```python
from build123d import *

# Parameters (mm, degrees)
BOSS_EXTRU_1_DEPTH      = 1380
ENL_V_MAT_EXTRU_1_DEPTH = 70


with BuildPart() as part:
    # Esquisse2 → Boss.-Extru.1 (new body)
    with BuildSketch(Plane.XY):
        with BuildLine():
            Line((2, 0), (38, 0))
            ThreePointArc((38, 0), (39.414213562, 0.585786438), (40, 2))
            Line((40, 2), (40, 38))
            ThreePointArc((40, 38), (39.414213562, 39.414213562), (38, 40))
            Line((38, 40), (2, 40))
            ThreePointArc((2, 40), (0.585786438, 39.414213562), (0, 38))
            Line((0, 38), (0, 2))
            ThreePointArc((0, 2), (0.585786438, 0.585786438), (2, 0))
        make_face()
        with BuildLine():
            Line((6, 4), (34, 4))
            ThreePointArc((34, 4), (35.414213562, 4.585786438), (36, 6))
            Line((36, 6), (36, 34))
            ThreePointArc((36, 34), (35.414213562, 35.414213562), (34, 36))
            Line((34, 36), (6, 36))
            ThreePointArc((6, 36), (4.585786438, 35.414213562), (4, 34))
            Line((4, 34), (4, 6))
            ThreePointArc((4, 6), (4.585786438, 4.585786438), (6, 4))
        make_face(mode=Mode.SUBTRACT)
    extrude(amount=BOSS_EXTRU_1_DEPTH)

    # Esquisse3 → Enlèv. mat.-Extru.1 (cut)
    with BuildSketch(Plane(origin=(0, 40, 0), x_dir=(1, 0, 0), z_dir=(0, 1, 0))):
        Polygon((0, -1380), (40, -1340), (40, -1380), align=None)
    extrude(amount=-ENL_V_MAT_EXTRU_1_DEPTH, mode=Mode.SUBTRACT)


solid = part.part
```
Check sheet for the modelled part. Datum: model origin and axes. Units: mm. A direction names the side the tool comes from. Give positions to 0.01 mm unless a question says otherwise; leave off trailing zeros. Order: outer loops, then holes, each group sorted by start corner. A loop starts at its lowest first (then second) coordinate and runs counter-clockwise, first axis right, second up. Notation, with made-up numbers: M 11.5,27.5 L 61.5,27.5 A33 ccw 61.5,58.5 Z; hole C 58,61.5 d5. An arc over 180 degrees is marked long. Answer in a Markdown table with one row per item.
1) Access from +Z, -Z, +X, -X, +Y, -Y to the whole of each face (thin tool, end or side, straight path). Record for faces 1 (the flat face through (4, 20, 678)), 2 (the flat face through (40, 20, 661)).
Filled sheet:
| item | result |
|---|---|
| face 1 | +Z, -Z |
| face 2 | +Z, -Z, +X, +Y, -Y |
2) Release check for a two-part mould opening along Y. For faces 3 (the flat face through (20, 4, 677)), 4 (the flat face through (36, 20, 663)), 5 (the flat face through (20, 0, 679)), 6 (the flat face through (20, 3, 1360)) record: +Y half, -Y half, draft (parallel to the pull), parting line (faces both ways), or undercut.
Filled sheet:
| item | result |
|---|---|
| face 3 | undercut |
| face 4 | undercut |
| face 5 | -Y half |
| face 6 | draft |
3) Thickness scan on L1, parallel to X at y = 6.5, z = 839.5; L2, parallel to Z at x = 2, y = 24.5. Record the ranges inside material, lowest first. Write a range as [from, to].
Filled sheet:
| item | result |
|---|---|
| L1 | x = [0, 4], [36, 40] |
| L2 | z = [0, 1378] |
4) Cross-section at A-A, the plane x = 17. Enter the section's corners in (y, z).
Filled sheet:
| item | result |
|---|---|
| outline | M 0,0 L 4,0 L 4,1363 L 0,1363 Z; M 36,0 L 40,0 L 40,1363 L 36,1363 Z |
5) Cross-section at B-B, the plane y = 19.5. Enter the section's corners in (x, z).
Filled sheet:
| item | result |
|---|---|
| outline | M 0,0 L 4,0 L 4,1376 L 0,1380 Z; M 36,0 L 40,0 L 40,1340 L 36,1344 Z |
6) Cross-section at C-C, the plane z = 1127.5. Enter the section's corners in (x, y), plus the area to 3 significant figures.
Filled sheet:
| item | result |
|---|---|
| outline | M 0,2 A2 ccw 2,0 L 38,0 A2 ccw 40,2 L 40,38 A2 ccw 38,40 L 2,40 A2 ccw 0,38 Z; hole M 4,6 A2 ccw 6,4 L 34,4 A2 ccw 36,6 L 36,34 A2 ccw 34,36 L 6,36 A2 ccw 4,34 Z |
| area | 576 mm2 |
7) Gauge pin test, flat end, axial feed: P1, Ø1.5, axis at x = 4.5, y = 20.5, coming from the +Z side. Record the tip position at first contact, or that the pin passes through.
Filled sheet:
| item | result |
|---|---|
| P1 | stops at z = 1376.25 |
